The model under review builds one solid part; all positions refer to its coordinate system, in mm. A direction names the side the tool comes from. Coordinates: 2 decimals unless noted, no trailing zeros. Loops run counter-clockwise (first coordinate to the right, second up) from the corner with the lowest first, then second, coordinate; pieces in that order, holes last. Notation, with made-up numbers: (27.25, 40) - (58.25, 40) arc R19 cw to (58.25, 63) - close; hole circle Ø7 at (32, 9.25). An arc over 180 degrees is marked (long way). One line per item, written item: value. Start each with the question number.
1. Insertion check: P1, Ø3.5, axis at x = -15.5, z = 5.5, coming from the -Y side; P2, Ø20, axis at x = -7, y = -6, coming from the +Z side; P3, Ø3, axis at x = -10, y = -23.5, coming from the +Z side; P4, Ø1, axis at x = -14.5, z = 11.5, coming from the +Y side. Each pin has a flat end and moves straight along its axis. Give the tip position at first contact, or say it passes through.
2. Mouldability with a two-part tool opening along X and no side actions: class faces 6 (the face through (-10.676, 0, 8)), 7 (the face through (15, 0, 13.54)), 8 (the face through (-18.551, -28.472, 1.288)) as +X half, -X half, draft (parallel to the pull), parting line (faces both ways), or undercut.
3. We need section A-A, the plane z = 7.75. Give the boundary of the cut face in (x, y).
4. For faces 1 (the face through (13.406, 5.624, 8.117)), 2 (the face through (-17.676, 0, 8)), 3 (the face through (11.604, -3, 8)), 4 (the face through (-14, -7.333, 8)), 5 (the face through (-14, 7.331, 8)), list the 3-axis set-ups (+Z, -Z, +X, -X, +Y, -Y) from which the entire face can be reached by the end or side of a thin tool; tool diameter is ignored.
5. We need section B-B, the plane x = -11.5. Give the boundary of the cut face in (y, z), then the cut area to 3 significant figures.
6. We need section C-C, the plane y = 0. Give the boundary of the cut face in (x, z), then the cut area to 3 significant figures.
7. To check wall thickness, follow line 1 (X direction, y = -0.5, z = 12.5); line 2 (Y direction, x = -14, z = 13.25); line 3 (Z direction, x = -7.5, y = -19.5). State the ranges of each line that lie inside material, in increasing order.
8. We need section D-D, the plane y = -12.5. Give the boundary of the cut face in (x, z).
from build123d import *

# Parameters (mm, degrees)
F0_W     = 40
F0_H     = 60
F1_DEPTH = 2.54
F2_R     = 5.08
F3_W     = 7
F3_H     = 14.663703
F4_DEPTH = 11
F5_R     = 5.991668


with BuildPart() as f1:
    # F0 (on Top) → F1 (new body)
    with BuildSketch(Plane.XY):
        Rectangle(F0_W, F0_H)
    extrude(amount=F1_DEPTH)

    # F2
    f2_edges = [f1.edges().sort_by_distance(p)[0] for p in [
        (-20, -30, 1.27),
        (20, -30, 1.27),
        (-20, 30, 1.27),
        (20, 30, 1.27),
    ]]
    fillet(f2_edges, radius=F2_R)

    # F3 (on face) → F4 (join)
    with BuildSketch(Plane.XY.offset(2.54)):
        Polygon((-17.676001, -7.332922), (-10.676001, -7.332922), (-10.676001, 7.330781), (-11.603794, 7.330781), (-17.676001, 7.330781), align=None)
        with Locations((15.103794, 0.00107)):
            Rectangle(F3_W, F3_H)
    extrude(amount=F4_DEPTH)

    # F5
    f5_edges = [f1.edges().sort_by_distance(p)[0] for p in [
        (11.603794, 7.332922, 8.04),
    ]]
    fillet(f5_edges, radius=F5_R)


solid = f1.part
Findings below:
1. P1: y = -7.33
1. P2: z = 13.54
1. P3: z = 2.54
1. P4: y = 7.33
2. face 6: undercut
2. face 7: draft
2. face 8: -X half
3. outline: (-17.68, -7.33) - (-10.68, -7.33) - (-10.68, 7.33) - (-17.68, 7.33) - close; (11.6, -7.33) - (18.6, -7.33) - (18.6, 7.33) - (17.6, 7.33) arc R5.99 ccw to (11.6, 1.34) - close
4. face 1: +Z, +Y
4. face 2: +Z, -X, +Y, -Y
4. face 3: +Z, +Y, -Y
4. face 4: +Z, +X, -X, -Y
4. face 5: +Z, +X, -X, +Y
5. outline: (-30, 0) - (30, 0) - (30, 2.54) - (7.33, 2.54) - (7.33, 13.54) - (-7.33, 13.54) - (-7.33, 2.54) - (-30, 2.54) - close
5. area: 314 mm2
6. outline: (-20, 0) - (20, 0) - (20, 2.54) - (18.6, 2.54) - (18.6, 13.54) - (11.6, 13.54) - (11.6, 2.54) - (-10.68, 2.54) - (-10.68, 13.54) - (-17.68, 13.54) - (-17.68, 2.54) - (-20, 2.54) - close
6. area: 256 mm2
7. line 1: -17.68 to -10.68, 11.6 to 18.6
7. line 2: -7.33 to 7.33
7. line 3: 0 to 2.54
8. outline: (-20, 0) - (20, 0) - (20, 2.54) - (-20, 2.54) - close
